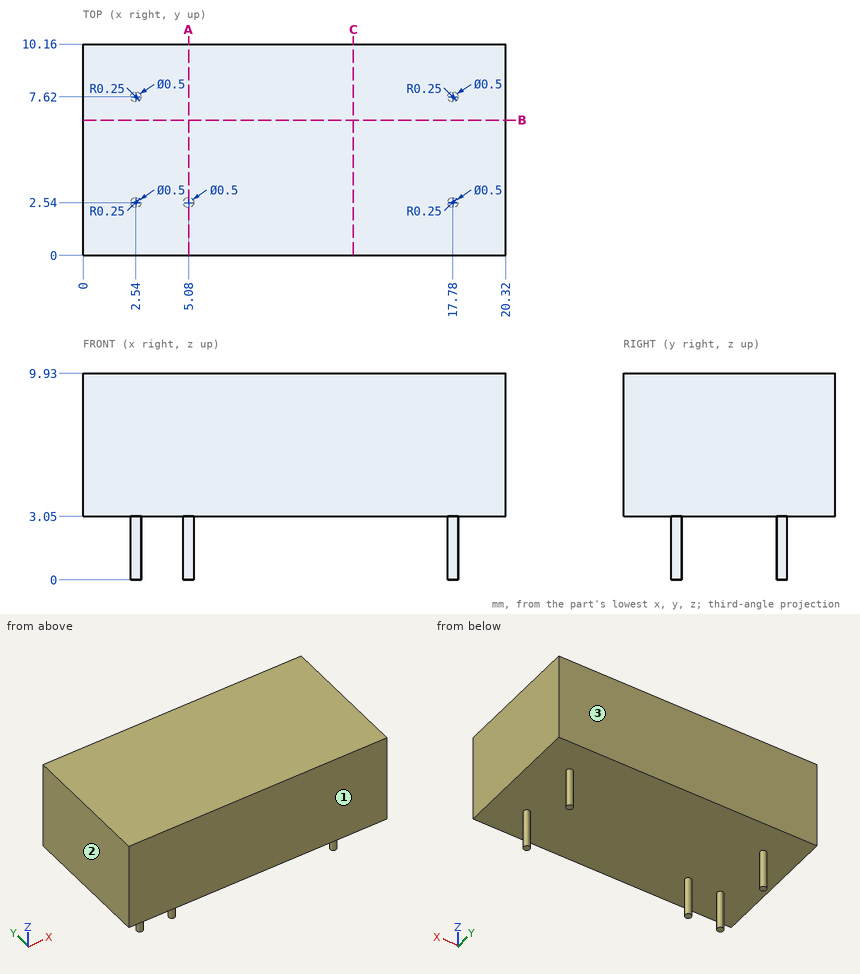
Input: dimensioned drawing with shaded views. Units: mm. Origin: part minimum x, y, z. Give positions to 0.01 mm unless a question says otherwise; leave off trailing zeros. Order: outer loops, then holes, each group sorted by start corner. A loop starts at its lowest first (then second) coordinate and runs counter-clockwise, first axis right, second up. Notation, with made-up numbers: (11, 70.25) -> (36, 70.25) arc R30 cw to (36, 101.25) -> close; hole circle Ø9 at (21.25, 21.25). An arc over 180 degrees is marked (long way). Use a Markdown table: item, result.
1) Ray query, line 1 along Z through (x, y) = (11.5, 0.5). Return the intervals inside material, ascending. Write a range as [from, to].
Answer list:
| item | result |
|---|---|
| line 1 | [3.05, 9.93] |
2) Section query B-B, the plane y = 6.5. Return the cut outline in (x, z).
Answer list:
| item | result |
|---|---|
| outline | (0, 3.05) -> (20.32, 3.05) -> (20.32, 9.93) -> (0, 9.93) -> close |
3) Section query C-C, the plane x = 13. Return the cut outline in (y, z), then the cut area to 3 significant figures.
Answer list:
| item | result |
|---|---|
| outline | (0, 3.05) -> (10.16, 3.05) -> (10.16, 9.93) -> (0, 9.93) -> close |
| area | 69.9 mm² |
4) Contact query for a flat-ended pin moving along its axis: P1, Ø3, axis at x = 13, y = 7.5, coming from the -Z side. Output: stop coordinate, or through.
Answer list:
| item | result |
|---|---|
| P1 | z = 3.05 |
5) Section query A-A, the plane x = 5.08. Return the cut outline in (y, z).
Answer list:
| item | result |
|---|---|
| outline | (0, 3.05) -> (2.29, 3.05) -> (2.29, 0) -> (2.79, 0) -> (2.79, 3.05) -> (10.16, 3.05) -> (10.16, 9.93) -> (0, 9.93) -> close |
6) Mould query, pull axis Y, two halves, no side actions, for the marked faces 1, 2 and 3. Classes: +Y half, -Y half, draft (parallel to the pull), parting line (faces both ways), or undercut.
Answer list:
| item | result |
|---|---|
| face 1 | -Y half |
| face 2 | draft |
| face 3 | +Y half |
